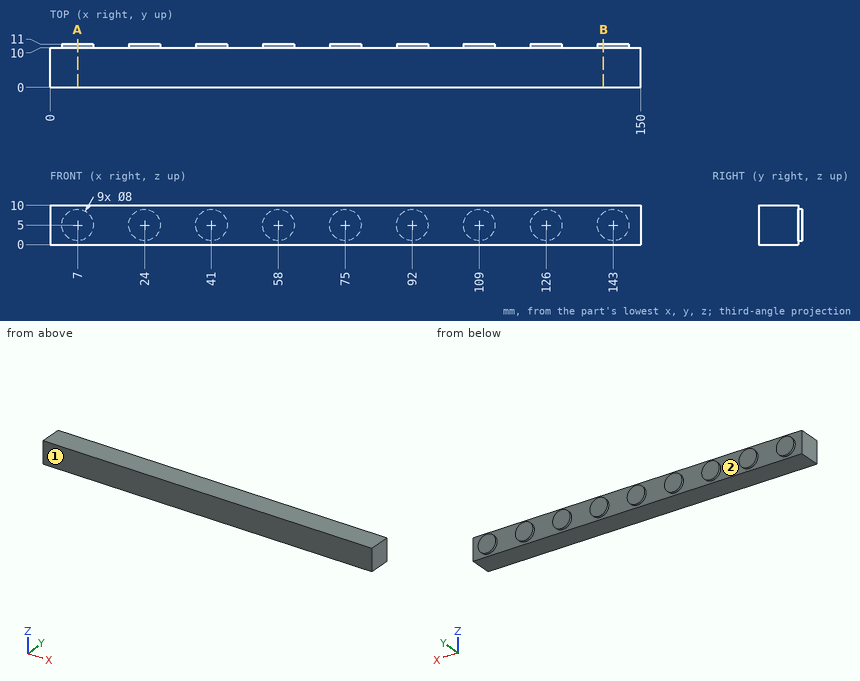
The figure shows three views and two pictorial views of one solid part (mm, origin at its lowest corner). Answer the questions. Round coordinates to 2 decimals unless told otherwise and drop trailing zeros. Write each loop counter-clockwise with the first axis right and the second up, starting at its lowest first coordinate (ties: lowest second). Pieces come first, ordered by that corner, then holes. Notation, with made-up numbers: (-23, 29.25) - (19, 29.25) arc R30 cw to (19, 60.25) - close; hole circle Ø3 at (-6, -8.5). An arc over 180 degrees is marked (long way). One line per question, with ' | ' between items. Start each with the question number.
1. Find the intervals of material crossed by probe 1 along Y at (x, z) = (68, 2.5); probe 2 along Z at (x, y) = (56, 10.75), in increasing order. Write a range as [from, to].
2. For a pull along X with two mould halves and no side action, classify the marked faces 1 and 2 as +X half, -X half, draft (parallel to the pull), parting line (faces both ways), or undercut.
3. Section B-B (x = 140.5) is taken. Determine the outline of the cut face in (y, z).
4. This flat-tipped pin is pushed along its axis until it touches: pin 1 (3 mm diameter, centred on x = 50.5, z = 7, fed in from +Y). Where does it stop, or does it pass through?
5. Section A-A (x = 7) is taken. Determine the outline of the cut face in (y, z).
Filled in:
1) probe 1: [0, 10] | probe 2: [1.54, 8.46]
2) face 1: draft | face 2: undercut
3) outline: (0, 0) - (10, 0) - (10, 1.88) - (11, 1.88) - (11, 8.12) - (10, 8.12) - (10, 10) - (0, 10) - close
4) pin 1: y = 10
5) outline: (0, 0) - (10, 0) - (10, 1) - (11, 1) - (11, 9) - (10, 9) - (10, 10) - (0, 10) - close
